Work out the finished part from the listing and answer in its coordinate system (mm). Face numbers are marked on the shaded views. A direction names the side the tool comes from. Coordinates: 2 decimals unless noted, no trailing zeros. Order: outer loops, then holes, each group sorted by start corner. A loop starts at its lowest first (then second) coordinate and runs counter-clockwise, first axis right, second up. Notation, with made-up numbers: M -26.5,-5.75 L 7.5,-5.75 A26 ccw 7.5,18.25 Z; hole C 4.5,4 d2. An arc over 180 degrees is marked long. Write item = value, one per line. Start each with the question number.
Q1. Find section A-A on y = 3.8. Give the vertices of the cut face in (x, z) (3 decimals).
Q2. Straight lines are drawn through the part: line 1 along Y through (x, z) = (-1.5, 0) (3 decimals); line 2 along X through (y, z) = (1.4, -1.75); line 3 along Z through (x, y) = (-1, 3.8) (3 decimals). For each, find the intervals that lie inside material, in ascending order.
Q3. Each of these flat-tipped pins is pushed along its axis until it touches: P1, Ø0.5, axis at y = 1, z = -1.5, coming from the +X side; P2, Ø0.5, axis at x = -2.5, z = 1, coming from the -Y side; P3, Ø1.6, axis at y = 0.5, z = -1, coming from the -X side; P4, Ø1.6, axis at y = 3.8, z = 0, coming from the +X side. Where does it stop, or does it pass through?
Q4. Find section B-B on z = 2.5. Give the vertices of the cut face in (x, y).
Q5. Find section C-C on x = 0. Give the vertices of the cut face in (y, z) (3 decimals).
Q6. Find section D-D on z = 0. Give the vertices of the cut face in (x, y) (3 decimals).
Q7. A tool of negligible diameter and unlimited length cuts with its end or side. For the marked faces 1, 2 and 3, from which of +Z, -Z, +X, -X, +Y, -Y can it reach the whole face along a straight path? Write none if from no direction.
Q8. Determine the mould class of the marked faces 4, 5, 6 and 7 for opening direction Z: released by +Z, released by -Z, zero draft, split by the parting line, or undercut.
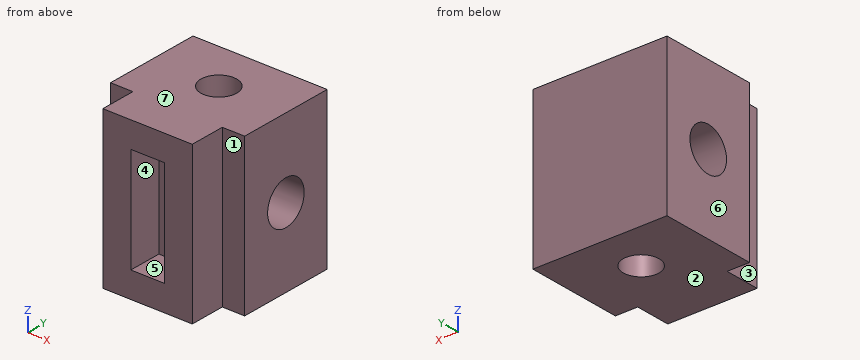
```python
from build123d import *

# Parameters (mm, degrees)
SKETCH1_W           = 4
SKETCH1_H           = 7
BOSS_EXTRUDE1_DEPTH = 6
SKETCH2_W           = 1.5
SKETCH2_H           = 4.7
CUT_EXTRUDE1_DEPTH  = 1.5
CUT_EXTRUDE2_REACH  = 9
SKETCH3_R           = 0.8
SKETCH5_W           = 1
SKETCH5_H           = 4.4
BOSS_EXTRUDE2_DEPTH = 7
SKETCH4_R           = 0.975
CUT_EXTRUDE4_DEPTH  = 7


with BuildPart() as part:
    # Sketch1 → Boss-Extrude1 (new body)
    with BuildSketch(Plane(origin=(0, 0, 0), x_dir=(1, 0, 0), z_dir=(0, 1, 0))):
        Rectangle(SKETCH1_W, SKETCH1_H)
    extrude(amount=BOSS_EXTRUDE1_DEPTH)

    # Sketch2 → Cut-Extrude1 (cut)
    with BuildSketch(Plane.XZ):
        Rectangle(SKETCH2_W, SKETCH2_H)
    extrude(amount=-CUT_EXTRUDE1_DEPTH, mode=Mode.SUBTRACT)

    # Sketch3 → Cut-Extrude2 (cut, up to next)
    with BuildSketch(Plane.XY.offset(3.5), mode=Mode.PRIVATE) as cut_extrude2_sk1:
        with Locations((0, 3.8)):
            Circle(SKETCH3_R)
    cut_extrude2_tool1 = extrude(cut_extrude2_sk1.sketch, amount=-CUT_EXTRUDE2_REACH, mode=Mode.PRIVATE) & part.part
    add(cut_extrude2_tool1.solids().sort_by_distance((0, 3.8, 3.5))[0], mode=Mode.SUBTRACT)

    # Sketch5 → Boss-Extrude2 (add)
    with BuildSketch(Plane.XY.offset(3.5)):
        with Locations((2.5, 3.8)):
            Rectangle(SKETCH5_W, SKETCH5_H)
        with Locations((-2.5, 3.8)):
            Rectangle(SKETCH5_W, SKETCH5_H)
    extrude(amount=-BOSS_EXTRUDE2_DEPTH)

    # Sketch4 → Cut-Extrude4 (cut, through all)
    with BuildSketch(Plane.ZY.offset(3)):
        with Locations((0, 3.8)):
            Circle(SKETCH4_R)
    extrude(amount=-CUT_EXTRUDE4_DEPTH, mode=Mode.SUBTRACT)


solid = part.part
```
Findings below:
q1.outline = M -3,-3.5 L -0.8,-3.5 L -0.8,-0.975 L -3,-0.975 Z; M -3,0.975 L -0.8,0.975 L -0.8,3.5 L -3,3.5 Z; M 0.8,-3.5 L 3,-3.5 L 3,-0.975 L 0.8,-0.975 Z; M 0.8,0.975 L 3,0.975 L 3,3.5 L 0.8,3.5 Z
q2.line_1 = 0 to 2.825, 4.775 to 6
q2.line_2 = -2 to -0.75, 0.75 to 2
q2.line_3 = -3.5 to -0.975, 0.975 to 3.5
q3.P1 = 2
q3.P2 = 1.6
q3.P3 = -2
q3.P4 = through
q4.outline = M -3,1.6 L -2,1.6 L -2,0 L 2,0 L 2,1.6 L 3,1.6 L 3,6 L -3,6 Z; hole C 0,3.8 d1.6
q5.outline = M 0,-3.5 L 3,-3.5 L 3,-0.557 A0.975 cw 3,0.557 L 3,3.5 L 0,3.5 L 0,2.35 L 1.5,2.35 L 1.5,-2.35 L 0,-2.35 Z; M 4.6,-3.5 L 6,-3.5 L 6,3.5 L 4.6,3.5 L 4.6,0.557 A0.975 cw 4.6,-0.557 Z
q6.outline = M -3,1.6 L -2,1.6 L -2,0 L -0.75,0 L -0.75,1.5 L 0.75,1.5 L 0.75,0 L 2,0 L 2,1.6 L 3,1.6 L 3,2.825 L -3,2.825 Z; M -3,4.775 L 3,4.775 L 3,6 L -3,6 Z
q7.face_1 = +Z, -Z, +X, -Y
q7.face_2 = -Z, +X, -X, +Y, -Y
q7.face_3 = +Z, -Z, -X, -Y
q8.face_4 = undercut
q8.face_5 = undercut
q8.face_6 = zero draft
q8.face_7 = released by +Z
